Could you check a few things on this model? Use its own coordinates, in mm. A direction names the side the tool comes from. Coordinates: 2 decimals unless noted, no trailing zeros. Write each loop counter-clockwise with the first axis right and the second up, starting at its lowest first coordinate (ties: lowest second). Pieces come first, ordered by that corner, then holes.
```python
from build123d import *

# Parameters (mm, degrees)
F0_R            = 18
F1_DEPTH        = 91
F2_R            = 11
F3_DEPTH        = 2
F4_R            = 4
F5_DEPTH        = 18
F6_R            = 1.5
F7_DEPTH        = 5
F7_COPIES_COUNT = 4
F9_START        = 5
F8_W            = 20
F8_H            = 10
F9_DEPTH        = 20


# Not quite as in the source:
# - a pattern or mirror of a feature is missing from the dataset's text; its kind, count and spacing are read off the source's solid


with BuildPart() as f1:
    # F0 (on Right) → F1 (new body)
    with BuildSketch(Plane.YZ):
        Circle(F0_R)
    extrude(amount=-F1_DEPTH)

    # F2 (on Right) → F3 (join)
    with BuildSketch(Plane.YZ):
        Circle(F2_R)
    extrude(amount=F3_DEPTH)

    # F4 (on Right) → F5 (join)
    with BuildSketch(Plane.YZ):
        Circle(F4_R)
    extrude(amount=F5_DEPTH)

    # F6 (on Right) → F7 (cut)
    with BuildSketch(Plane.YZ):
        with Locations((14, 0)):
            Circle(F6_R)
    f7 = extrude(amount=-F7_DEPTH, mode=Mode.SUBTRACT)

    # F7_copies: F7 ×4 about axis
    f7_copies_axis = Axis((0, 0, 0), (1, 0, 0))
    for i in range(1, F7_COPIES_COUNT):
        add(f7.rotate(f7_copies_axis, i * 360 / F7_COPIES_COUNT), mode=Mode.SUBTRACT)

    # F8 (on Right) → F9 (cut)
    with BuildSketch(Plane.YZ.offset(F9_START)):
        with Locations((0, -8)):
            Rectangle(F8_W, F8_H)
    extrude(amount=F9_DEPTH, mode=Mode.SUBTRACT)


solid = f1.part
```
1. I want a section at B-B on z = 0. Please give me the cut outline in (x, y), plus the area to 3 significant figures.
Verdict:
outline: (-91, -18) - (0, -18) - (0, -15.5) - (-5, -15.5) - (-5, -12.5) - (0, -12.5) - (0, -11) - (2, -11) - (2, -4) - (18, -4) - (18, 4) - (2, 4) - (2, 11) - (0, 11) - (0, 12.5) - (-5, 12.5) - (-5, 15.5) - (0, 15.5) - (0, 18) - (-91, 18) - close
area: 3,420 mm2
2. Please list where these lines run through material, in increasing order: line 1 along X through (y, z) = (1.5, 12); line 2 along Z through (x, y) = (-32.5, 0.5); line 3 along X through (y, z) = (0.5, 7.5).
Verdict:
line 1: x = -91 to 0
line 2: z = -17.99 to 17.99
line 3: x = -91 to 2
3. For pin 1 (12 mm diameter, centred on x = -23, z = -8.5, fed in from -Y); pin 2 (2.5 mm diameter, centred on x = 8.5, y = 1, fed in from -Z); pin 3 (4 mm diameter, centred on y = -14, z = 0, fed in from +X), each with a flat end and sliding along its axis, tell me the tip position at first contact or that it passes through.
Verdict:
pin 1: stops at y = -17.83
pin 2: stops at z = -3
pin 3: stops at x = 0
4. I want a section at C-C on x = -33. Please give me the cut outline in (y, z), plus the area to 3 significant figures.
Verdict:
outline: circle Ø36 at (0, 0)
area: 1,020 mm2
5. I want a section at A-A on y = 0. Please give me the cut outline in (x, z).
Verdict:
outline: (-91, -18) - (0, -18) - (0, -15.5) - (-5, -15.5) - (-5, -12.5) - (0, -12.5) - (0, -11) - (2, -11) - (2, -4) - (5, -4) - (5, -3) - (18, -3) - (18, 4) - (2, 4) - (2, 11) - (0, 11) - (0, 12.5) - (-5, 12.5) - (-5, 15.5) - (0, 15.5) - (0, 18) - (-91, 18) - close
6. I want a section at D-D on z = -14. Please give me the cut outline in (x, y), plus the area to 3 significant figures.
Verdict:
outline: (-91, -11.31) - (0, -11.31) - (0, -1.5) - (-5, -1.5) - (-5, 1.5) - (0, 1.5) - (0, 11.31) - (-91, 11.31) - close
area: 2,040 mm2
7. If we mould it in two halves opening along Y, with no side actions, what happens to faces 1 (the face through (11, 0, -3)), 2 (the face through (9.888, -0.521, 3.966)), 3 (the face through (-2.46, 0.07, -12.5))? For each: pulls with the +Y half, pulls with the -Y half, needs draft (parallel to the pull), parting line crosses it, or undercut.
Verdict:
face 1: needs draft
face 2: parting line crosses it
face 3: undercut
8. On a 3-axis mill with a long thin cutter (end or side, diameter ignored), from which of +Z, -Z, +X, -X, +Y, -Y can I reach the whole of each face in a straight line? I mean faces 4 (the face through (18, 0, 1)), 5 (the face through (-5, 0, -14)). Say none if no direction works.
Verdict:
face 4: +Z, -Z, +X, +Y, -Y
face 5: +X
